Geometry check sheet. Reference: the model listing, model coordinates, mm. A direction names the side the tool comes from. Give positions to 0.01 mm unless a question says otherwise; leave off trailing zeros. Write each loop counter-clockwise with the first axis right and the second up, starting at its lowest first coordinate (ties: lowest second). Pieces come first, ordered by that corner, then holes. Notation, with made-up numbers: (-3.75, 39) - (32.25, 39) arc R17 cw to (32.25, 67) - close; hole circle Ø5 at (-40, 27). An arc over 180 degrees is marked (long way). Write item = value, one per line. Start each with the question number.
(1) Access from +Z, -Z, +X, -X, +Y, -Y to the whole of each face (thin tool, end or side, straight path). Record for faces 5 (the flat face through (-1, -15, -200)), 6 (the flat face through (0, -7, -150)).
(2) Section check B-B, the plane y = -12. Enter the section's corners in (x, z), plus the area to 3 significant figures.
(3) Section check D-D, the plane z = -8. Enter the section's corners in (x, y), plus the area to 3 significant figures.
(4) Thickness scan on L1, parallel to Z at x = 2, y = -8.5; L2, parallel to X at y = -11, z = -118; L3, parallel to Z at x = 9, y = -13.5. Record the ranges inside material, lowest first.
(5) Section check A-A, the plane x = 0. Enter the section's corners in (y, z).
(6) Draft check along X on faces 1 (the flat face through (-50, -7, -125)), 2 (the flat face through (50, -7, -125)), 3 (the flat face through (29, -7, 2)), 4 (the flat face through (-1, 0, -200)). Enter one of: pulls with the +X half, pulls with the -X half, needs draft (parallel to the pull), parting line crosses it, or undercut.
(7) Section check C-C, the plane x = 36. Enter the section's corners in (y, z).
```python
from build123d import *

# Parameters (mm, degrees)
SKETCH1_W               = 100
SKETCH1_H               = 600
BOSS_EXTRUDE2_DEPTH     = 15
SKETCH1_7_W             = 58
SKETCH1_7_H             = 300
CUT_EXTRUDE1_DEPTH      = 65
SKETCH1_8_R             = 45
CUT_EXTRUDE2_DEPTH      = 433.1643206
CUT_EXTRUDE4_DEPTH      = 441.195695118
CUT_EXTRUDE4_DEPTH_BACK = 441.195695118


with BuildPart() as part:
    # Sketch1 → Boss-Extrude2 (new body)
    with BuildSketch(Plane(origin=(0, 0, 0), x_dir=(1, 0, 0), z_dir=(0, 1, 0))):
        with Locations((0, 129)):
            Rectangle(SKETCH1_W, SKETCH1_H)
    extrude(amount=-BOSS_EXTRUDE2_DEPTH)

    # Sketch1<7> → Cut-Extrude1 (cut)
    with BuildSketch(Plane(origin=(0, 0, 0), x_dir=(1, 0, 0), z_dir=(0, 1, 0))):
        Rectangle(SKETCH1_7_W, SKETCH1_7_H)
    extrude(amount=-CUT_EXTRUDE1_DEPTH, mode=Mode.SUBTRACT)

    # Sketch1<8> → Cut-Extrude2 (cut, through all)
    with BuildSketch(Plane(origin=(0, 0, 0), x_dir=(1, 0, 0), z_dir=(0, 1, 0))):
        with Locations(Location((0, 344, 0), (0, 0, 270))):
            Circle(SKETCH1_8_R)
    extrude(amount=-CUT_EXTRUDE2_DEPTH, mode=Mode.SUBTRACT)

    # Sketch5 → Cut-Extrude4 (cut, two sides: drawn at the far end of the back side and taken through both)
    with BuildSketch(Plane(origin=(47.5, 0, 0), x_dir=(0, 0, -1), z_dir=(1, 0, 0)).offset(-CUT_EXTRUDE4_DEPTH_BACK)):
        with BuildLine():
            ThreePointArc((346, -7.5), (345.414213562, -6.085786438), (344, -5.5))
            Line((344, -5.5), (344, -9.5))
            ThreePointArc((344, -9.5), (345.414213562, -8.914213562), (346, -7.5))
        make_face()
        with BuildLine():
            Line((344, -9.5), (344, -5.5))
            ThreePointArc((344, -5.5), (342, -7.5), (344, -9.5))
        make_face()
    extrude(amount=CUT_EXTRUDE4_DEPTH + CUT_EXTRUDE4_DEPTH_BACK, mode=Mode.SUBTRACT)


solid = part.part
```
Model answer:
q1.face_5 = +Z, -Z, +X, -X, -Y
q1.face_6 = +Y, -Y
q2.outline = (-50, -429) - (50, -429) - (50, 171) - (-50, 171) - close; hole circle Ø90 at (0, -344); hole (-29, -150) - (29, -150) - (29, 150) - (-29, 150) - close
q2.area = 36,200 mm²
q3.outline = (-50, -15) - (-29, -15) - (-29, 0) - (-50, 0) - close; (29, -15) - (50, -15) - (50, 0) - (29, 0) - close
q3.area = 630 mm²
q4.L1 = -429 to -388.96, -299.04 to -150, 150 to 171
q4.L2 = -50 to -29, 29 to 50
q4.L3 = -429 to -388.09, -299.91 to -150, 150 to 171
q5.outline = (-15, -429) - (0, -429) - (0, -389) - (-15, -389) - close; (-15, -299) - (0, -299) - (0, -150) - (-15, -150) - close; (-15, 150) - (0, 150) - (0, 171) - (-15, 171) - close
q6.face_1 = pulls with the -X half
q6.face_2 = pulls with the +X half
q6.face_3 = undercut
q6.face_4 = needs draft
q7.outline = (-15, -429) - (0, -429) - (0, -371) - (-15, -371) - close; (-15, -317) - (0, -317) - (0, 171) - (-15, 171) - close
